```python
from build123d import *

# Parameters (mm, degrees)
F0_W      = 69.85
F0_H      = 38.1
F1_DEPTH  = 25.4
F5_DEPTH  = 50.8
F7_DEPTH  = 25.4
F8_R      = 6.35
F9_DEPTH  = 50.8
F11_DEPTH = 25.4
F13_DEPTH = 25.4


# Not quite as in the source:
# - a feature of the source that left no trace in its solid (it failed there, or was rolled back) is left out


with BuildPart() as f1:
    # F0 (on Front) → F1 (new body)
    with BuildSketch(Plane.XZ):
        with Locations((34.925, 19.05)):
            Rectangle(F0_W, F0_H)
    extrude(amount=F1_DEPTH)

    # F4 (on face) → F5 (cut)
    with BuildSketch(Plane.XY.offset(38.1)):
        with BuildLine():
            ThreePointArc((0, -12.7), (3.7197438789, -3.7197438789), (12.7, 0))
            Line((12.7, 0), (0, 0))
            Line((0, 0), (0, -12.7))
        make_face()
        with BuildLine():
            Line((0, -25.4), (12.7, -25.4))
            ThreePointArc((12.7, -25.4), (3.7197438789, -21.6802561211), (0, -12.7))
            Line((0, -12.7), (0, -25.4))
        make_face()
    extrude(amount=-F5_DEPTH, mode=Mode.SUBTRACT)

    # F6 (on face) → F7 (cut)
    with BuildSketch(Plane.XY.offset(38.1)):
        with BuildLine():
            ThreePointArc((12.7, 0), (25.4, -12.7), (12.7, -25.4))
            Line((12.7, -25.4), (69.85, -25.4))
            Line((69.85, -25.4), (69.85, 0))
            Line((69.85, 0), (12.7, 0))
        make_face()
    extrude(amount=-F7_DEPTH, mode=Mode.SUBTRACT)

    # F8 (on face) → F9 (cut)
    with BuildSketch(Plane.XY.offset(38.1)):
        with Locations((12.7, -12.7)):
            Circle(F8_R)
    extrude(amount=-F9_DEPTH, mode=Mode.SUBTRACT)

    # F10 (on face) → F11 (cut)
    with BuildSketch(Plane.XY.offset(12.7)):
        with BuildLine():
            ThreePointArc((38.1, -19.05), (42.5901280605, -17.1901280605), (44.45, -12.7))
            ThreePointArc((44.45, -12.7), (42.7995135722, -8.4295114817), (38.7060402567, -6.37898622))
            Line((38.7060402567, -6.37898622), (38.1, -19.05))
        make_face()
        with BuildLine():
            ThreePointArc((38.7060402567, -6.37898622), (42.7995135722, -8.4295114817), (44.45, -12.7))
            ThreePointArc((44.45, -12.7), (42.5901280605, -17.1901280605), (38.1, -19.05))
            Line((38.1, -19.05), (57.15, -19.05))
            ThreePointArc((57.15, -19.05), (50.8000019615, -12.7049911232), (57.1400177568, -6.3500078461))
            Line((57.1400177568, -6.3500078461), (38.7060402567, -6.37898622))
        make_face()
        with BuildLine():
            Line((38.1, -19.05), (38.7060402567, -6.37898622))
            ThreePointArc((38.7060402567, -6.37898622), (31.7572506946, -12.3966334751), (38.1, -19.05))
        make_face()
        with BuildLine():
            Line((57.15, -19.05), (57.1400177568, -6.3500078461))
            ThreePointArc((57.1400177568, -6.3500078461), (50.8000019615, -12.7049911232), (57.15, -19.05))
        make_face()
        with BuildLine():
            ThreePointArc((63.5, -12.7), (61.6365974165, -8.2063440694), (57.1400177568, -6.3500078461))
            Line((57.1400177568, -6.3500078461), (57.15, -19.05))
            ThreePointArc((57.15, -19.05), (61.6401280605, -17.1901280605), (63.5, -12.7))
        make_face()
    extrude(amount=-F11_DEPTH, mode=Mode.SUBTRACT)

    # F12 (on face) → F13 (cut)
    with BuildSketch(Plane.XY.offset(12.7)):
        with BuildLine():
            ThreePointArc((58.1890903413, 0), (68.7523295615, -13.1579480832), (57.1400177568, -25.4))
            Line((57.1400177568, -25.4), (69.85, -25.4))
            Line((69.85, -25.4), (69.85, 0))
            Line((69.85, 0), (58.1890903413, 0))
        make_face()
    extrude(amount=-F13_DEPTH, mode=Mode.SUBTRACT)


solid = f1.part
```
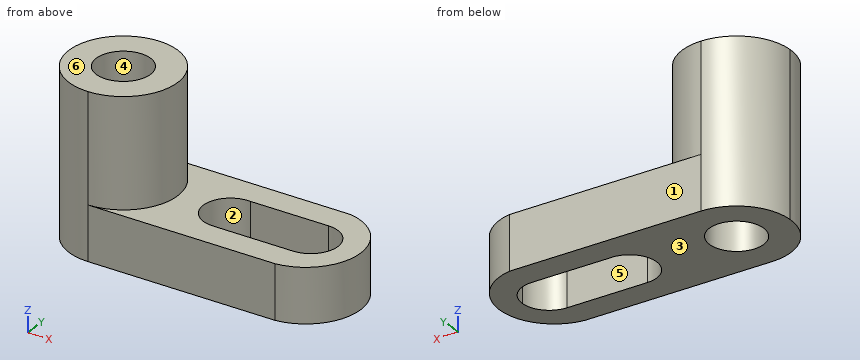
Verification items for the finished model (mm, model axes). Face numbers are marked on the shaded views. A direction names the side the tool comes from. Round coordinates to 2 decimals unless told otherwise and drop trailing zeros. Loops run counter-clockwise (first coordinate to the right, second up) from the corner with the lowest first, then second, coordinate; pieces in that order, holes last. Notation, with made-up numbers: (83, -4.75) -> (133, -4.75) arc R17 ccw to (133, 22.25) -> close; hole circle Ø6 at (33.25, 29). An arc over 180 degrees is marked (long way). Answer as a JSON object with one key per item and string values.
Q1. Section check A-A (x = 10). Record the boundary of the cut face in (y, z), then the cut area to 3 significant figures.
Data:
{"outline": "(-25.11, 0) -> (-18.45, 0) -> (-18.45, 38.1) -> (-25.11, 38.1) -> close; (-6.95, 0) -> (-0.29, 0) -> (-0.29, 38.1) -> (-6.95, 38.1) -> close", "area": "508 mm2"}
Q2. Section check D-D (x = 21.5). Record the boundary of the cut face in (y, z).
Data:
{"outline": "(-25.4, 0) -> (0, 0) -> (0, 12.7) -> (-3.54, 12.7) -> (-3.54, 38.1) -> (-21.86, 38.1) -> (-21.86, 12.7) -> (-25.4, 12.7) -> close"}
Q3. Draft check along Y on the marked faces 1, 2, 3 and 4. Enter one of: pulls with the +Y half, pulls with the -Y half, needs draft (parallel to the pull), parting line crosses it, or undercut.
Data:
{"face 1": "pulls with the +Y half", "face 2": "undercut", "face 3": "needs draft", "face 4": "undercut"}
Q4. Access from +Z, -Z, +X, -X, +Y, -Y to the whole of each face (thin tool, end or side, straight path). Record for the marked faces 5 and 6.
Data:
{"face 5": "+Z, -Z", "face 6": "+Z, +X, -X, +Y, -Y"}
Q5. Section check C-C (z = 20). Record the boundary of the cut face in (x, y), then the cut area to 3 significant figures.
Data:
{"outline": "circle Ø25.4 at (12.7, -12.7); hole circle Ø12.7 at (12.7, -12.7)", "area": "380 mm2"}
Q6. Section check B-B (y = -10.25). Record the boundary of the cut face in (x, z).
Data:
{"outline": "(0.24, 0) -> (6.84, 0) -> (6.84, 38.1) -> (0.24, 38.1) -> close; (18.56, 0) -> (32.24, 0) -> (32.24, 12.7) -> (25.16, 12.7) -> (25.16, 38.1) -> (18.56, 38.1) -> close; (63.01, 0) -> (68.54, 0) -> (68.54, 12.7) -> (63.01, 12.7) -> close"}
Q7. Scan lines: line 1 (X direction, y = -8.75, z = 8.5); line 2 (Y direction, x = 40, z = 2.5); line 3 (Z direction, x = 63, y = -4.75). Record each from-to range of solid material in increasing order. Write a range as from..to.
Data:
{"line 1": "x = 0.63..7.73, 17.67..33.13, 62.12..68.16", "line 2": "y = -25.4..-19.05, -6.38..0", "line 3": "z = 0..12.7"}
Q8. Go/stop test with flat-tipped pins: P1, Ø12, axis at x = 24.5, z = 31.5, coming from the -Y side; P2, Ø5, axis at y = -10.5, z = 19.5, coming from the +X side; P3, Ø12, axis at y = -3, z = 9.5, coming from the -X side; P4, Ø7.5, axis at x = 12.7, y = -12.7, coming from the +Z side. Record where each tip stops, or that it passes through.
Data:
{"P1": "stops at y = -24", "P2": "stops at x = 25.4", "P3": "stops at x = 0.55", "P4": "passes through"}
